Can you work these out from the model? Positions are in its coordinate system, mm. A direction names the side the tool comes from. Coordinates: 2 decimals unless noted, no trailing zeros. Write each loop counter-clockwise with the first axis right and the second up, starting at its lowest first coordinate (ties: lowest second). Pieces come first, ordered by that corner, then holes. Notation, with made-up numbers: (-4, -39.5) - (10, -39.5) arc R29 ccw to (10, -16.5) - close; hole circle Ø2 at (0, 64.5). An arc over 180 degrees is marked (long way). Use one line per item in the form item = value. Start each with the question number.
(1) Thinking about a two-plate mould opening in Y: for faces 1 (the face through (-49, -26.254, 49)), 2 (the face through (64.969, -1, 49)), 3 (the face through (-18.734, -30.402, 49.3)), 4 (the face through (-62, 28.596, 49)), which applies, pulls with the +Y half, pulls with the -Y half, needs draft (parallel to the pull), parting line crosses it, or undercut?
(2) If I drill on probe 1 along Y at (x, z) = (64, 62.5); probe 2 along Y at (x, z) = (-50, 59); probe 3 along Y at (x, z) = (28, 46), over which ranges is the centre line in solid material (lowest first)? Write a range as from..to.
(3) On a 3-axis mill with a long thin cutter (end or side, diameter ignored), from which of +Z, -Z, +X, -X, +Y, -Y can I reach the whole of each face in a straight line? I mean faces 5 (the face through (64.969, -36, 49)), 6 (the face through (-53.031, 7, 49)), 7 (the face through (-61, 30.596, 49)), 8 (the face through (-55.031, -1, 49)), 9 (the face through (20, -12, 0)). Say none if no direction works.
(4) If we section it at A-A on y = 16: Give the number of separate pieces and of enclosed holes in the cut face, then the cut area to 3 significant figures.
(5) For pin 1 Ø1.2 at (y, z) = (-34, 56) entering from -X; pin 2 Ø3 at (x, z) = (-63, 30) entering from -Y; pin 3 Ø2.5 at (y, z) = (-31.5, 68.5) entering from -X; pin 4 Ø1 at (x, y) = (33.5, -10.5) entering from -Z, each with a flat end and sliding along its axis, tell me the tip position at first contact or that it passes through.
(6) If we section it at B-B on x = 46.5: Please give me the cut outline in (y, z), then the cut area to 3 significant figures.
```python
from build123d import *

# Parameters (mm, degrees)
PAD_DEPTH = 100


with BuildPart() as part:
    # Sketch002 → Pad (new body)
    with BuildSketch(Plane.XY):
        with BuildLine():
            Line((64.96916, -39.403533), (64.96916, -33.053533))
            Line((64.96916, -33.053533), (61.96916, -33.053533))
            Line((61.96916, -33.053533), (61.96916, -34.553533))
            Line((61.96916, -34.553533), (56.96916, -34.553533))
            Line((56.96916, -30.403533), (56.96916, -34.553533))
            Line((56.96916, -26.253533), (56.96916, -30.403533))
            Line((56.96916, -26.253533), (61.96916, -26.253533))
            Line((61.96916, -26.253533), (61.96916, -27.753533))
            Line((61.96916, -27.753533), (64.96916, -27.753533))
            Line((64.96916, -27.753533), (64.96916, 26.596467))
            ThreePointArc((66.96916, 28.596467), (65.554946, 28.010681), (64.96916, 26.596467))
            Line((66.96916, 28.596467), (77.46916, 28.596467))
            Line((77.46916, 28.596467), (77.46916, 30.596467))
            Line((77.46916, 30.596467), (64.96916, 30.596467))
            ThreePointArc((64.96916, 30.596467), (63.554946, 30.010681), (62.96916, 28.596467))
            Line((62.96916, 28.596467), (62.96916, -15.403533))
            ThreePointArc((54.96916, -15.403533), (58.96916, -19.403533), (62.96916, -15.403533))
            Line((54.96916, -15.403533), (53.16916, 29.346467))
            ThreePointArc((53.16916, 29.346467), (52.112017, 30.40361), (51.054874, 29.346467))
            Line((51.054874, 29.346467), (50.254874, -24.403533))
            ThreePointArc((38.254874, -24.403533), (44.254874, -30.403533), (50.254874, -24.403533))
            Line((38.254874, -24.403533), (37.454874, 29.346467))
            ThreePointArc((37.454874, 29.346467), (36.397731, 30.40361), (35.340589, 29.346467))
            Line((35.340589, 29.346467), (34.540589, -24.403533))
            ThreePointArc((22.540589, -24.403533), (28.540589, -30.403533), (34.540589, -24.403533))
            Line((22.540589, -24.403533), (21.740589, 29.346467))
            ThreePointArc((21.740589, 29.346467), (20.683446, 30.40361), (19.626303, 29.346467))
            Line((19.626303, 29.346467), (18.826303, -24.403533))
            ThreePointArc((6.826303, -24.403533), (12.826303, -30.403533), (18.826303, -24.403533))
            Line((6.826303, -24.403533), (6.026303, 29.346467))
            ThreePointArc((6.026303, 29.346467), (4.96916, 30.40361), (3.912017, 29.346467))
            Line((3.112017, -24.403533), (3.912017, 29.346467))
            ThreePointArc((-8.887983, -24.403533), (-2.887983, -30.403533), (3.112017, -24.403533))
            Line((-9.687983, 29.346467), (-8.887983, -24.403533))
            ThreePointArc((-9.687983, 29.346467), (-10.745126, 30.40361), (-11.802269, 29.346467))
            Line((-12.602269, -24.403533), (-11.802269, 29.346467))
            ThreePointArc((-24.602269, -24.403533), (-18.602269, -30.403533), (-12.602269, -24.403533))
            Line((-25.402269, 29.346467), (-24.602269, -24.403533))
            ThreePointArc((-25.402269, 29.346467), (-26.459411, 30.40361), (-27.516554, 29.346467))
            Line((-28.316554, -24.403533), (-27.516554, 29.346467))
            ThreePointArc((-40.316554, -24.403533), (-34.316554, -30.403533), (-28.316554, -24.403533))
            Line((-41.116554, 29.346467), (-40.316554, -24.403533))
            ThreePointArc((-41.116554, 29.346467), (-42.173697, 30.40361), (-43.23084, 29.346467))
            Line((-45.03084, -15.403533), (-43.23084, 29.346467))
            ThreePointArc((-53.03084, -15.403533), (-49.03084, -19.403533), (-45.03084, -15.403533))
            Line((-53.03084, 28.596467), (-53.03084, -15.403533))
            ThreePointArc((-53.03084, 28.596467), (-53.616626, 30.010681), (-55.03084, 30.596467))
            Line((-67.53084, 30.596467), (-55.03084, 30.596467))
            Line((-67.53084, 28.596467), (-67.53084, 30.596467))
            Line((-57.03084, 28.596467), (-67.53084, 28.596467))
            ThreePointArc((-55.03084, 26.596467), (-55.616626, 28.010681), (-57.03084, 28.596467))
            Line((-55.03084, -27.753533), (-55.03084, 26.596467))
            Line((-52.03084, -27.753533), (-55.03084, -27.753533))
            Line((-52.03084, -26.253533), (-52.03084, -27.753533))
            Line((-47.03084, -26.253533), (-52.03084, -26.253533))
            Line((-47.03084, -26.253533), (-47.03084, -30.403533))
            Line((-47.03084, -30.403533), (-47.03084, -34.553533))
            Line((-52.03084, -34.553533), (-47.03084, -34.553533))
            Line((-52.03084, -33.053533), (-52.03084, -34.553533))
            Line((-55.03084, -33.053533), (-52.03084, -33.053533))
            Line((-55.03084, -39.403533), (-55.03084, -33.053533))
            Line((64.96916, -39.403533), (-55.03084, -39.403533))
        make_face()
    extrude(amount=PAD_DEPTH)


solid = part.part
```
Reported:
q1.face_1 = undercut
q1.face_2 = needs draft
q1.face_3 = pulls with the +Y half
q1.face_4 = pulls with the -Y half
q2.probe_1 = -39.4..-33.05, -27.75..30.35
q2.probe_2 = -39.4..-34.55, -26.25..-19.28
q2.probe_3 = -39.4..-30.38
q3.face_5 = +Z, -Z, +X, -Y
q3.face_6 = +Z, -Z, +Y
q3.face_7 = +Z, -Z, +X, -X, +Y
q3.face_8 = +Z, -Z, -X, -Y
q3.face_9 = -Z, +X, -X, +Y, -Y
q4.separate_pieces = 9
q4.enclosed_holes = 0
q4.area = 2,230 mm2
q5.pin_1 = -55.03
q5.pin_2 = 28.6
q5.pin_3 = -47.03
q5.pin_4 = through
q6.outline = (-39.4, 0) - (-29.97, 0) - (-29.97, 100) - (-39.4, 100) - close
q6.area = 944 mm2
